Geometry: final body of the model. Coordinates: model frame, mm. A direction names the side the tool comes from. Give positions to 0.01 mm unless a question says otherwise; leave off trailing zeros. Loops run counter-clockwise (first coordinate to the right, second up) from the corner with the lowest first, then second, coordinate; pieces in that order, holes last. Notation, with made-up numbers: (-20, 71.25) - (1, 71.25) arc R12 ccw to (1, 81.25) - close; hole circle Ø3 at (51.25, 13). An arc over 180 degrees is marked (long way). Use one line per item in the form item = value.
Autodesk Inventor part; units mm, degrees
ref_plane "YZ Plane" through (0, 0, 0) normal (1, 0, 0) x (0, 1, 0)
ref_plane "XZ Plane" through (0, 0, 0) normal (0, 1, 0) x (-1, 0, 0)
ref_plane "XY Plane" through (0, 0, 0) normal (0, 0, 1) x (1, 0, 0)
sketch "Sketch1" plane through (0, 0, 0) normal (1, 0, 0) x (0, 1, 0)
  line L0 (0, 0) -> (11.176, 0)
  line L1 (11.176, -22.098) -> (0, -22.098)
  line L2 (0, -22.098) -> (0, 0)
  line L3 (11.176, 0) -> (11.176, -5.5245)
  line L4 (11.176, -22.098) -> (11.176, -16.5735)
  line L5 (11.176, -5.5245) -> (15.494, -5.5245)
  line L6 (15.494, -5.5245) -> (15.494, -16.5735)
  line L7 (15.494, -16.5735) -> (11.176, -16.5735)
  line L8 (11.176, 0) -> (11.176, -5.5245)
  line L9 (11.176, -16.5735) -> (11.176, -22.098)
  dimension "d0" = 11.176
  dimension "d1" = 22.098
  dimension "d2" = 5.5245
  dimension "d3" = 5.5245
  dimension "d4" = 4.318
extrude "Extrusion1" add sketch "Sketch1" along normal blind 1.524
sketch "Sketch2" plane through (1.524, 0, 0) normal (1, 0, 0) x (0, 0, -1)
  line L0 (16.5735, 15.494) -> (5.5245, 15.494)
  line L1 (5.5245, 13.97) -> (16.5735, 13.97)
  line L2 (16.5735, 11.176) -> (16.5735, 15.494)
  line L3 (16.5735, 13.97) -> (21.9075, 13.97)
  line L4 (21.9075, 13.97) -> (21.9075, 15.494)
  line L5 (21.9075, 15.494) -> (16.5735, 15.494)
  line L6 (5.5245, 15.494) -> (0.1905, 15.494)
  line L7 (0.1905, 15.494) -> (0.1905, 13.97)
  line L8 (0.1905, 13.97) -> (5.5245, 13.97)
  point P0 (0, 0)
extrude "Extrusion2" add sketch "Sketch2" along normal blind 30.734
fillet "Fillet1" radius 1.27 1 edges at (0, 15.494, -11.049)
fillet "Fillet2" radius 0.254 1 edges at (1.524, 13.97, -11.049)
sketch "Sketch3" plane through (1.524, 0, 0) normal (1, 0, 0) x (0, 0, -1)
  line L0 (22.098, 0) -> (22.098, 11.176)
  line L1 (0, 0) -> (22.098, 0)
  circle A0 centre (19.558, 2.54) radius 1.397
  line L2 (22.098, 11.176) -> (16.5735, 11.176)
  circle A1 centre (19.558, 8.636) radius 1.397
  circle A2 centre (2.54, 2.54) radius 1.397
  circle A3 centre (2.54, 8.636) radius 1.397
  line L3 (11.049, 1.524) -> (11.049, 12.446) construction
  line L4 (12.573, 3.048) -> (12.573, 10.922)
  line L5 (9.525, 10.922) -> (9.525, 3.048)
  arc A4 (9.525, 3.048) -> (12.573, 3.048) centre (11.049, 3.048) ccw
  arc A5 (12.573, 10.922) -> (9.525, 10.922) centre (11.049, 10.922) ccw
  point P0 (11.049, 6.985)
  dimension "d16" = 2.794
  dimension "d19" = 2.794
  dimension "d23" = 10.922
  dimension "d24" = 3.048
  dimension "d50" = 17.018
extrude "Extrusion3" cut sketch "Sketch3" against normal blind 30.734
sketch "Sketch4" plane through (1.524, 15.494, -0.1905) normal (0, 1, 0) x (1, 0, 0)
  line L0 (-1.524, 16.383) -> (0, 16.383)
  line L1 (0, 16.383) -> (7.112, 16.383)
  line L2 (-0.254, 5.334) -> (0, 5.334)
  line L3 (0, 5.334) -> (7.112, 5.334)
  line L4 (7.112, 16.383) -> (7.112, 21.717)
  line L5 (0, 21.717) -> (30.734, 21.717)
  line L6 (7.112, 21.717) -> (0, 21.717)
  line L7 (0, 21.9075) -> (0, 16.383)
  line L8 (0, 21.717) -> (0, 16.383)
  line L9 (7.112, 5.334) -> (7.112, 0)
  line L10 (0, 0) -> (30.734, 0)
  line L11 (7.112, 0) -> (0, 0)
  line L12 (0, 5.334) -> (0, 16.383)
  line L13 (0, 0) -> (0, 5.334)
  point P0 (-1.524, -0.1905)
  dimension "d27" = 7.112
  dimension "d28" = 7.112
extrude "Extrusion4" cut sketch "Sketch4" against normal blind 30.734
sketch "Sketch5" plane through (32.258, 13.97, -21.9075) normal (0, -1, 0) x (1, 0, 0)
  circle A0 centre (-11.811, 10.8585) radius 5.08
  line L0 (-23.622, 21.717) -> (0, 21.717)
  circle A1 centre (-11.811, 21.717) radius 5.08
  line L1 (-23.622, 0) -> (0, 0)
  circle A2 centre (-11.811, 0) radius 5.08
  point P0 (-32.258, 21.9075)
  dimension "d31" = 10.16
  dimension "d32" = 10.16
  dimension "d33" = 10.16
extrude "Extrusion5" cut sketch "Sketch5" against normal blind 30.734
sketch "Sketch6" plane through (32.258, 13.97, -21.9075) normal (0, -1, 0) x (1, 0, 0)
  circle A0 centre (-2.032, 19.685) radius 1.397
  circle A1 centre (-11.811, 10.8585) radius 5.08
  line L0 (0, 21.717) -> (0, 0)
  line L1 (0, 0) -> (0, 2.032)
  line L2 (0, 2.032) -> (-2.032, 2.032)
  circle A2 centre (-2.032, 2.032) radius 1.397
  line L3 (-23.622, 21.717) -> (-23.622, 16.383)
  line L4 (-23.622, 21.717) -> (-23.622, 19.685)
  line L5 (-23.622, 19.685) -> (-21.59, 19.685)
  circle A3 centre (-21.59, 19.685) radius 1.397
  line L6 (-23.622, 5.334) -> (-23.622, 0)
  line L7 (-23.622, 0) -> (-23.622, 2.032)
  line L8 (-23.622, 2.032) -> (-21.59, 2.032)
  circle A4 centre (-21.59, 2.032) radius 1.397
  point P0 (-32.258, 21.9075)
  dimension "d38" = 2.794
  dimension "d39" = 2.032
  dimension "d40" = 2.032
  dimension "d41" = 2.794
  dimension "d42" = 2.032
  dimension "d43" = 2.032
  dimension "d44" = 2.794
  dimension "d45" = 2.032
  dimension "d46" = 2.032
  dimension "d47" = 2.794
extrude "Extrusion6" cut sketch "Sketch6" against normal blind 25.4 contours A0 | A2 | A3 | A4
properties part number "msheehan_motor_mount"
(1) Pin query (flat end, axial travel): P1, Ø1.5, axis at y = 2, z = -13.5, coming from the -X side; P2, Ø4.5, axis at x = 5.5, y = 13, coming from the -Z side; P3, Ø4, axis at y = 5, z = -11, coming from the +X side; P4, Ø0.8, axis at x = 13.5, y = 15, coming from the -Z side. Return the tip coordinate at first contact, or that it passes through.
Solution:
P1 = 0
P2 = -16.57
P3 = 1.52
P4 = -21.91
(2) Access query for faces 5 (the face through (13, 13.97, -11)), 6 (the face through (3.3, 14.3, -16.574)), 7 (the face through (8.636, 15, -19)). Directions: +Z, -Z, +X, -X, +Y, -Y. A direction counts if a zero-diameter tool reaches every point of the face in a straight line with its end or side. Return the directions, or none.
Solution:
face_5 = +Z, -Z, +X, -Y
face_6 = -Z, -X, +Y
face_7 = -Z, -X, +Y, -Y
(3) Material intervals for L1, parallel to Y at x = 0.6, z = -2.54; L2, parallel to X at y = 2.5, z = -17.5; L3, parallel to Y at x = 28, z = -7.5, sorted ascending. Write a range as from..to.
Solution:
L1 = 0..1.14, 3.94..7.24, 10.03..11.18
L2 = 0..1.52
L3 = 13.97..15.49
(4) Cut plane A-A (y = 4.75). Return the cut outline in (x, z) (3 decimals), plus the area to 3 significant figures.
Solution:
outline = (0, -22.098) - (1.524, -22.098) - (1.524, -12.573) - (0, -12.573) - close; (0, -9.525) - (1.524, -9.525) - (1.524, 0) - (0, 0) - close
area = 29.0 mm2
(5) Cut plane C-C (z = -10.25). Return the cut outline in (x, y).
Solution:
outline = (0, 0) - (1.52, 0) - (1.52, 1.75) - (0, 1.75) - close; (0, 12.22) - (1.52, 12.22) - (1.52, 13.72) arc R0.25 cw to (1.78, 13.97) - (15.43, 13.97) - (15.43, 15.49) - (1.27, 15.49) arc R1.27 ccw to (0, 14.22) - close; (25.46, 13.97) - (32.26, 13.97) - (32.26, 15.49) - (25.46, 15.49) - close
(6) Cut plane B-B (x = 11). Return the cut outline in (y, z).
Solution:
outline = (13.97, -21.91) - (15.49, -21.91) - (15.49, -21.23) - (13.97, -21.23) - close; (13.97, -18.52) - (15.49, -18.52) - (15.49, -3.58) - (13.97, -3.58) - close; (13.97, -0.87) - (15.49, -0.87) - (15.49, -0.19) - (13.97, -0.19) - close
(7) Cut plane D-D (x = 25). Return the cut outline in (y, z), plus the area to 3 significant figures.
Solution:
outline = (13.97, -19.65) - (15.49, -19.65) - (15.49, -13.3) - (13.97, -13.3) - close; (13.97, -8.8) - (15.49, -8.8) - (15.49, -2.44) - (13.97, -2.44) - close
area = 19.4 mm2
(8) Pull-direction query (Y, two-part tool) for faces 1 (the face through (0.773, 7.397, -3.185)), 2 (the face through (0.77, 2.96, -20.89)), 3 (the face through (1, 0, -11)), 4 (the face through (8.636, 15, -3)); classes: released by +Y, released by -Y, zero draft, split by the parting line, or undercut.
Solution:
face_1 = undercut
face_2 = undercut
face_3 = released by -Y
face_4 = zero draft
